Geometry check sheet. Reference: the model listing, model coordinates, mm. A direction names the side the tool comes from. Round coordinates to 2 decimals unless told otherwise and drop trailing zeros. Write each loop counter-clockwise with the first axis right and the second up, starting at its lowest first coordinate (ties: lowest second). Pieces come first, ordered by that corner, then holes. Notation, with made-up numbers: M -7,66 L 16,66 A25 cw 16,103 Z; hole C 58.25,52 d7. An arc over 180 degrees is marked long. One line per item, written item: value. Start each with the question number.
1. Access from +Z, -Z, +X, -X, +Y, -Y to the whole of each face (thin tool, end or side, straight path). Record for faces 5 (the flat face through (-13, 4, 2)), 6 (the flat face through (-40, -10, 3)), 7 (the flat face through (-16, 4, 0)), 8 (the flat face through (-21, 11, 7.25)).
2. Section check B-B (y = 17.5). Record the boundary of the cut face in (x, z).
3. Section check A-A (x = -49.9). Record the boundary of the cut face in (y, z) (3 decimals), and give its area (3 significant figures).
4. Section check C-C (z = 14.25). Record the boundary of the cut face in (x, y).
5. Scan lines: probe 1 along Y at (x, z) = (-2.1, 5.75); probe 2 along Z at (x, y) = (-49.9, -6.65) (3 decimals). Record each from-to range of solid material in increasing order. Write a range as [from, to].
6. Release check for a two-part mould opening along Y. For faces 1 (the flat face through (-25.2, 17, 5)), 2 (the cylindrical face through (-22.05, 9.97, 3.57)), 3 (the flat face through (-26.5, 11, 4)), 4 (the flat face through (-13, 26.5, 4)) record: pulls with the +Y half, pulls with the -Y half, needs draft (parallel to the pull), parting line crosses it, or undercut.
7. Depth check by flat-ended pin: P1, Ø3, axis at y = -0.5, z = -2, coming from the +X side; P2, Ø6, axis at y = 0, z = 4, coming from the -X side; P3, Ø1.5, axis at x = -16, y = -7.5, coming from the +Z side; P4, Ø3, axis at x = -23.1, y = 22.8, coming from the +Z side. Enter the tip coordinate at first touch or a pass-through.
Autodesk Inventor part; units mm, degrees
ref_plane "YZ Plane" through (0, 0, 0) normal (1, 0, 0) x (0, 1, 0)
ref_plane "XZ Plane" through (0, 0, 0) normal (0, 1, 0) x (-1, 0, 0)
ref_plane "XY Plane" through (0, 0, 0) normal (0, 0, 1) x (1, 0, 0)
sketch "Sketch1" plane through (0, 0, 0) normal (0, 0, 1) x (1, 0, 0)
  line L0 (0, 0) -> (-25, 0)
  line L1 (-25, 25) -> (0, 25)
  line L2 (0, 25) -> (0, 0)
  circle A0 centre (-23.1, 22.7984) radius 1.1
  circle A1 centre (-2.1, 22.8) radius 1.1
  circle A2 centre (-23.1, 10.2984) radius 1.1
  circle A3 centre (-2.1, 10.3) radius 1.1
  line L3 (-25, 0) -> (-25.2, 0)
  line L4 (-25.2, 0) -> (-25.2, 25)
  line L5 (-25.2, 25) -> (-25, 25)
  dimension "d2" = 2.2
  dimension "d5" = 2.2
  dimension "d7" = 12.5
  dimension "d8" = 2.2
  dimension "d9" = 2.2
  dimension "d14" = 12.5
  dimension "d31" = 2.1
  dimension "d46" = 0.2
  dimension "d47" = 2.1
  dimension "d48" = 2.1
extrude "Base" add sketch "Sketch1" along normal blind 2
sketch "Sketch2" plane through (0, 0, 2) normal (0, 0, 1) x (1, 0, 0)
  line L0 (-26.5, 0) -> (-26.5, 26.5)
  line L1 (-26.5, 26.5) -> (1.5, 26.5)
  line L2 (1.5, 26.5) -> (1.5, 0)
  line L3 (1.5, 0) -> (0, 0)
  line L4 (0, 25) -> (-25.2, 25)
  line L5 (0, 0) -> (0, 25)
  line L6 (-25.2, 25) -> (-25.2, 0)
  line L7 (-25.2, 0) -> (-26.5, 0)
  point P0 (-25, 25)
  point P1 (-25, 0)
  dimension "d16" = 26.5
  dimension "d17" = 28
extrude "Walls" add sketch "Sketch2" along normal blind 5.25 and the other way blind 2
sketch "Sketch3" plane through (0, 0, 2) normal (0, 0, 1) x (1, 0, 0)
  circle A0 centre (-23.1, 10.2984) radius 1.1
  circle A1 centre (-23.1, 10.2984) radius 1.6
  circle A2 centre (-2.1, 10.3) radius 1.1
  circle A3 centre (-2.1, 10.3) radius 1.6
  circle A4 centre (-23.1, 22.7984) radius 1.1
  circle A5 centre (-23.1, 22.7984) radius 1.6
  circle A6 centre (-2.1, 22.8) radius 1.1
  circle A7 centre (-2.1, 22.8) radius 1.6
  point P0 (0, 0)
  dimension "d22" = 3.2
  dimension "d23" = 3.2
  dimension "d24" = 3.2
  dimension "d25" = 3.2
extrude "Spacers" add sketch "Sketch3" along normal up to surface (5.25 mm away)
sketch "Sketch4" plane through (0, 0, 2) normal (0, 0, 1) x (1, 0, 0)
  circle A0 centre (-23.1, 10.2984) radius 1.1
  arc A1 (-23.1938, 7.55) -> (-23.1, 13.0484) centre (-23.1, 10.2984) ccw
  circle A2 centre (-2.1, 10.3) radius 1.1
  arc A3 (-2.1, 13.05) -> (-2.1, 7.55) centre (-2.1, 10.3) ccw
  circle A4 centre (-23.1, 22.7984) radius 1.1
  circle A5 centre (-2.1, 22.8) radius 1.1
  line L0 (-4.85, 22.8) -> (-4.85, 25)
  line L1 (-25.2, 25) -> (0, 25)
  line L2 (-2.1, 20.05) -> (0, 20.05)
  line L3 (0, 25) -> (0, 0)
  line L4 (-2.1, 13.05) -> (0, 13.05)
  line L5 (-2.1, 7.55) -> (0, 7.55)
  line L6 (-23.1, 13.0484) -> (-25.2, 13.0484)
  line L7 (-23.1938, 7.55) -> (-25, 7.55)
  arc A6 (-4.85, 22.8) -> (-2.1, 20.05) centre (-2.1, 22.8) ccw
  line L8 (-25, 7.55) -> (-25.2, 7.55)
  line L9 (-25.2, 13.0484) -> (-25.2, 13.0484)
  line L10 (-25.2, 25) -> (-25.2, 0)
  line L11 (-25.2, 20.0484) -> (-25.2, 20.0484)
  line L12 (-20.35, 22.7984) -> (-20.35, 25.6874)
  line L13 (-23.1, 20.0484) -> (-25.85, 20.0484)
  arc A7 (-23.1, 20.0484) -> (-20.35, 22.7984) centre (-23.1, 22.7984) ccw
  point P0 (-25, 25)
  point P1 (-20.35, 25)
  point P2 (-25.2, 20.0484)
  dimension "d33" = 5.5
  dimension "d34" = 5.5
extrude "Spacer blocks" add sketch "Sketch4" along normal up to surface (5.25 mm away)
sketch "Sketch5" plane through (0, 0, 0) normal (0, 0, -1) x (-1, 0, 0)
  line L0 (-1.5, 26.5) -> (-1.5, 0)
  circle A0 centre (12.4, 10.3) radius 4.5
  point P0 (0, 0)
  dimension "d39" = 13.9
  dimension "d40" = 9
extrude "Camera Hole" cut sketch "Sketch5" against normal through all
fillet "Outside Fillet - 2mm" radius 2 1 edges at (-7.9, 10.3, 0)
fillet "Inside Fillet - 1mm" radius 0.5 2 edges at (-7.9, 10.3, 1.9999) (-7.9, 10.3, 2)
chamfer "Chamfer1" distance 0.5 angle 45 5 edges at (1.5, 13.25, 0) (1.5, 26.5, 3.625) (-12.5, 26.5, 0) (-26.5, 26.5, 3.625) (-26.5, 13.25, 0)
sketch "Sketch6" plane through (-25.2, 0, 2) normal (0, -1, 0) x (1, 0, 0)
  line L0 (-0.8, -2) -> (-1.3, -1.5)
  line L1 (26.2, -2) -> (-0.8, -2)
  line L2 (26.7, -1.5) -> (26.2, -2)
  line L3 (26.7, -1.5) -> (26.7, 5.25)
  line L4 (25.2, 5.25) -> (26.7, 5.25)
  line L5 (25.2, 0) -> (25.2, 5.25)
  line L6 (0, 0) -> (25.2, 0)
  line L7 (0, 0) -> (0, 5.25)
  line L8 (-1.3, 5.25) -> (0, 5.25)
  line L9 (-1.3, -1.5) -> (-1.3, 5.25)
  point P0 (25.2, -2)
extrude "Bottom Extension" add sketch "Sketch6" along normal blind 5
sketch "Sketch7" plane through (-25.2, -5, 2) normal (0, -1, 0) x (1, 0, 0)
  line L0 (26.7, 5.25) -> (25.2, 5.25)
  line L1 (26.7, 5.25) -> (20.1, 5.25)
  line L2 (20.1, 5.25) -> (20.1, -2)
  line L3 (26.7, 5.25) -> (25.2, 5.25) construction
  line L4 (25.2, 5.25) -> (25.2, 0) construction
  line L5 (25.2, 0) -> (0, 0) construction
  line L6 (0, 0) -> (0, 5.25) construction
  line L7 (0, 5.25) -> (-1.3, 5.25) construction
  line L8 (-1.3, 5.25) -> (-1.3, -1.5) construction
  line L9 (-1.3, -1.5) -> (-0.8, -2) construction
  line L10 (-0.8, -2) -> (26.2, -2) construction
  line L11 (26.2, -2) -> (26.7, -1.5) construction
  line L12 (26.7, -1.5) -> (26.7, 5.25) construction
  line L13 (20.1, -2) -> (-0.8, -2)
  line L14 (-1.3, -1.5) -> (-0.8, -2)
  line L15 (-1.3, -1.5) -> (-1.3, 5.25)
  line L16 (-1.3, 5.25) -> (0, 5.25)
  line L17 (0, 5.25) -> (5.3, 5.25)
  line L18 (5.3, 5.25) -> (5.3, 0)
  line L19 (5.3, 0) -> (20.1, 0)
  line L20 (5.3, 0) -> (5.3, 2.5)
  line L21 (5.3, 2.5) -> (20.1, 2.5)
  line L22 (26.7, 5.25) -> (26.7, -1.5)
  line L23 (26.2, -2) -> (26.7, -1.5)
  line L24 (20.1, -2) -> (26.2, -2)
  line L25 (5.3, 5.25) -> (-24.7, 5.25)
  line L26 (-24.7, 5.25) -> (-24.7, -2)
  line L27 (-24.7, -2) -> (-0.8, -2)
  point P0 (25.2, -2)
  point P1 (50.1, 5.25)
  dimension "d54" = 6.6
  dimension "d58" = 5.3
  dimension "d59" = 2.5
  dimension "d68" = 30
extrude "Mounting Arm" add sketch "Sketch7" along normal blind 5
sketch "Sketch10" plane through (-25.2, -5, 2) normal (0, 1, 0) x (1, 0, 0)
  line L0 (-24.7, -5.25) -> (-24.7, 2)
  circle A0 centre (-24.7, -1.625) radius 15
  point P0 (25.2, 2)
  dimension "d69" = 30
extrude "Extrusion10" add sketch "Sketch10" against normal blind 5
sketch "Sketch11" plane through (-25.2, -5, 2) normal (0, 1, 0) x (1, 0, 0)
  arc A0 (-10.1446, 2) -> (-10.1446, -5.25) centre (-24.7, -1.625) ccw
  circle A1 centre (-24.7, -1.625) radius 3
  point P0 (25.2, 2)
  dimension "d72" = 6
extrude "Extrusion11" cut sketch "Sketch11" against normal through all
fillet "Fillet6" radius 2.5 2 edges at (-35.3446, -7.5, 7.25) (-35.3446, -7.5, 0)
properties part number "Top R_3DPrint"
Result sheet:
1. face 5: +Z
1. face 6: +Z, -Z, +X, -X, -Y
1. face 7: -Z, +X, +Y, -Y
1. face 8: +Z, +X, +Y, -Y
2. outline: M -26.5,0.5 L -26,0 L 1,0 L 1.5,0.5 L 1.5,7.25 L 0,7.25 L 0,2 L -25.2,2 L -25.2,7.25 L -26.5,7.25 Z
3. outline: M -10,-11.375 L -5,-11.375 L -5,0.625 L -10,0.625 Z; M -10,6.625 L -5,6.625 L -5,18.625 L -10,18.625 Z
3. area: 120 mm2
4. outline: M -60.49,-10 L -39.31,-10 L -39.31,-5 L -60.49,-5 Z
5. probe 1: y = [-10, -5], [7.55, 9.2], [11.4, 13.05], [20.05, 21.7], [23.9, 26.5]
5. probe 2: z = [-11.375, 0.625], [6.625, 18.625]
6. face 1: undercut
6. face 2: undercut
6. face 3: needs draft
6. face 4: pulls with the +Y half
7. P1: passes through
7. P2: stops at x = -26.5
7. P3: stops at z = 4.5
7. P4: stops at z = 7.25
